For this review, take the finished solid that the model builds, in its own axes (mm). Give positions to 0.01 mm unless a question says otherwise; leave off trailing zeros. Loops run counter-clockwise (first coordinate to the right, second up) from the corner with the lowest first, then second, coordinate; pieces in that order, holes last.
Autodesk Inventor part; units mm, degrees
ref_plane "YZ Plane" through (0, 0, 0) normal (1, 0, 0) x (0, 1, 0)
ref_plane "XZ Plane" through (0, 0, 0) normal (0, 1, 0) x (-1, 0, 0)
ref_plane "XY Plane" through (0, 0, 0) normal (0, 0, 1) x (1, 0, 0)
sketch "スケッチ1" plane through (0, 0, 0) normal (0, 0, 1) x (1, 0, 0)
  line L0 (-70, 75) -> (70, 75)
  line L1 (70, 75) -> (70, -75)
  line L2 (70, -75) -> (-70, -75)
  line L3 (-70, -75) -> (-70, 75)
  line L4 (70, 92.6777) -> (87.6777, 75)
  line L5 (87.6777, 75) -> (70, 57.3223)
  line L6 (70, 57.3223) -> (52.3223, 75)
  line L7 (52.3223, 75) -> (70, 92.6777)
  line L8 (70, -57.3223) -> (87.6777, -75)
  line L9 (87.6777, -75) -> (70, -92.6777)
  line L10 (70, -92.6777) -> (52.3223, -75)
  line L11 (52.3223, -75) -> (70, -57.3223)
  line L12 (-70, -57.3223) -> (-52.3223, -75)
  line L13 (-52.3223, -75) -> (-70, -92.6777)
  line L14 (-70, -92.6777) -> (-87.6777, -75)
  line L15 (-87.6777, -75) -> (-70, -57.3223)
  line L16 (-70, 92.6777) -> (-52.3223, 75)
  line L17 (-52.3223, 75) -> (-70, 57.3223)
  line L18 (-70, 57.3223) -> (-87.6777, 75)
  line L19 (-87.6777, 75) -> (-70, 92.6777)
  point P0 (0, 0)
  point P1 (70, 75)
  dimension "d0" = 150
  dimension "d1" = 75
  dimension "d2" = 140
  dimension "d3" = 70
  dimension "d4" = 12.5
  dimension "d5" = 12.5
  dimension "d6" = 12.5
  dimension "d7" = 12.5
extrude "押し出し1" add sketch "スケッチ1" along normal blind 3
sketch "スケッチ2" plane through (0, 0, 3) normal (0, 0, 1) x (1, 0, 0)
  line L0 (87.6777, 75) -> (70, 57.3223)
  line L1 (70, 92.6777) -> (87.6777, 75)
  line L2 (52.3223, 75) -> (70, 92.6777)
  line L3 (-70, 92.6777) -> (-52.3223, 75)
  line L4 (-87.6777, 75) -> (-70, 92.6777)
  line L5 (-70, 57.3223) -> (-87.6777, 75)
  line L6 (-87.6777, -75) -> (-70, -57.3223)
  line L7 (-70, -92.6777) -> (-87.6777, -75)
  line L8 (-52.3223, -75) -> (-70, -92.6777)
  line L9 (70, -92.6777) -> (52.3223, -75)
  line L10 (87.6777, -75) -> (70, -92.6777)
  line L11 (70, -57.3223) -> (87.6777, -75)
  circle A0 centre (-56.2114, -49.8977) radius 1.5
  circle A1 centre (-44.8977, -61.2114) radius 1.5
  circle A2 centre (44.8977, -61.2114) radius 1.5
  circle A3 centre (56.2114, -49.8977) radius 1.5
  circle A4 centre (56.2114, 49.8977) radius 1.5
  circle A5 centre (44.8977, 61.2114) radius 1.5
  circle A6 centre (-44.8977, 61.2114) radius 1.5
  circle A7 centre (-56.2114, 49.8977) radius 1.5
  point P0 (0, 0)
  dimension "d10" = 3
  dimension "d12" = 40
  dimension "d13" = 40
  dimension "d14" = 4.5
  dimension "d15" = 4.5
  dimension "d16" = 40
  dimension "d17" = 40
  dimension "d18" = 40
  dimension "d19" = 40
  dimension "d20" = 40
  dimension "d21" = 40
  dimension "d22" = 4.5
  dimension "d23" = 4.5
  dimension "d24" = 4.5
  dimension "d25" = 4.5
  dimension "d26" = 4.5
  dimension "d27" = 4.5
hole "穴1" at (44.8977, -61.2114, 3) at (56.2114, -49.8977, 3) at (-44.8977, -61.2114, 3) at (-56.2114, -49.8977, 3) at (44.8977, 61.2114, 3) at (56.2114, 49.8977, 3) at (-56.2114, 49.8977, 3) at (-44.8977, 61.2114, 3) direction (0, 0, -1) diameter 3 end through all
sketch "スケッチ3" plane through (0, 0, 3) normal (0, 0, 1) x (1, 0, 0)
  line L0 (87.6777, 75) -> (70, 57.3223)
  line L1 (70, 92.6777) -> (87.6777, 75)
  line L2 (52.3223, 75) -> (70, 92.6777)
  line L3 (-70, 92.6777) -> (-52.3223, 75)
  line L4 (-87.6777, 75) -> (-70, 92.6777)
  line L5 (-70, 57.3223) -> (-87.6777, 75)
  line L6 (-87.6777, -75) -> (-70, -57.3223)
  line L7 (-70, -92.6777) -> (-87.6777, -75)
  line L8 (-52.3223, -75) -> (-70, -92.6777)
  line L9 (70, -92.6777) -> (52.3223, -75)
  line L10 (87.6777, -75) -> (70, -92.6777)
  line L11 (70, -57.3223) -> (87.6777, -75)
  circle A0 centre (-49.1403, 65.4541) radius 2.25
  circle A1 centre (-60.4541, 54.1403) radius 2.25
  circle A2 centre (-60.4541, -54.1403) radius 2.25
  circle A3 centre (-49.1403, -65.4541) radius 2.25
  circle A4 centre (49.1403, -65.4541) radius 2.25
  circle A5 centre (60.4541, -54.1403) radius 2.25
  circle A6 centre (60.4541, 54.1403) radius 2.25
  circle A7 centre (49.1403, 65.4541) radius 2.25
  point P0 (0, 0)
  dimension "d35" = 4.5
  dimension "d37" = 4.5
  dimension "d38" = 4.5
  dimension "d39" = 34
  dimension "d40" = 34
  dimension "d41" = 4.5
  dimension "d42" = 4.5
  dimension "d43" = 34
  dimension "d44" = 34
  dimension "d45" = 34
  dimension "d46" = 4.5
  dimension "d47" = 4.5
  dimension "d48" = 34
  dimension "d49" = 34
  dimension "d50" = 34
  dimension "d51" = 4.5
  dimension "d52" = 4.5
hole "穴2" at (-60.4541, -54.1403, 3) at (-49.1403, -65.4541, 3) at (49.1403, 65.4541, 3) at (60.4541, 54.1403, 3) at (-60.4541, 54.1403, 3) at (-49.1403, 65.4541, 3) at (49.1403, -65.4541, 3) at (60.4541, -54.1403, 3) direction (0, 0, -1) diameter 4.5 end through all
sketch "スケッチ4" plane through (0, 0, 3) normal (0, 0, 1) x (1, 0, 0)
  line L0 (87.6777, 75) -> (70, 57.3223)
  line L1 (70, 92.6777) -> (87.6777, 75)
  line L2 (52.3223, 75) -> (70, 92.6777)
  line L3 (-70, 92.6777) -> (-52.3223, 75)
  line L4 (-87.6777, 75) -> (-70, 92.6777)
  line L5 (-70, 57.3223) -> (-87.6777, 75)
  line L6 (-87.6777, -75) -> (-70, -57.3223)
  line L7 (-70, -92.6777) -> (-87.6777, -75)
  line L8 (-52.3223, -75) -> (-70, -92.6777)
  line L9 (70, -92.6777) -> (52.3223, -75)
  line L10 (87.6777, -75) -> (70, -92.6777)
  line L11 (70, -57.3223) -> (87.6777, -75)
  line L12 (-70, -57.3223) -> (-52.3223, -75)
  line L13 (52.3223, -75) -> (70, -57.3223)
  line L14 (52.3223, 75) -> (70, 57.3223)
  line L15 (-70, 57.3223) -> (-52.3223, 75)
  point P0 (0, 0)
  dimension "d60" = 25
  dimension "d61" = 25
  dimension "d62" = 25
  dimension "d63" = 25
extrude "押し出し2" cut sketch "スケッチ4" against normal blind 3
sketch "スケッチ6" plane through (-52.3223, 75, 0) normal (0, 1, 0) x (1, 0, 0)
  line L0 (104.6447, 0) -> (0, 0)
  line L1 (0, -3) -> (104.6447, -3)
  line L2 (39.8223, 0) -> (64.8223, 0)
  line L3 (64.8223, 0) -> (64.8223, -3)
  line L4 (64.8223, -3) -> (39.8223, -3)
  line L5 (39.8223, -3) -> (39.8223, 0)
  point P0 (52.3223, 0)
  dimension "d66" = 25
  dimension "d68" = 12.5
extrude "押し出し3" add sketch "スケッチ6" along normal blind 10
sketch "スケッチ7" plane through (0, 0, 3) normal (0, 0, 1) x (1, 0, 0)
  line L0 (-12.5, 85) -> (12.5, 85)
  line L1 (-12.5, 75) -> (-12.5, 85)
  circle A0 centre (-8, 73) radius 1.5
  circle A1 centre (8, 73) radius 1.5
  point P0 (0, 0)
  dimension "d71" = 16
  dimension "d72" = 12
  dimension "d73" = 12
  dimension "d74" = 3
  dimension "d75" = 4.5
hole "穴3" at (-8, 73, 3) at (8, 73, 3) direction (0, 0, -1) diameter 3 end through all
sketch "スケッチ9" plane through (0, 0, 3) normal (0, 0, 1) x (1, 0, 0)
  line L0 (52.3223, -75) -> (-52.3223, -75)
  circle A0 centre (-32.5, -61.5) radius 1.5
  circle A1 centre (-32.5, -28.5) radius 1.5
  circle A2 centre (-32.5, 4.5) radius 1.5
  circle A3 centre (32.5, -61.5) radius 1.5
  circle A4 centre (32.5, -28.5) radius 1.5
  circle A5 centre (32.5, 4.5) radius 1.5
  point P0 (0, 0)
  dimension "d95" = 3
  dimension "d97" = 13.5
  dimension "d98" = 33
  dimension "d99" = 33
  dimension "d100" = 33
  dimension "d101" = 33
  dimension "d102" = 13.5
  dimension "d103" = 65
  dimension "d104" = 65
  dimension "d105" = 65
  dimension "d106" = 32.5
  dimension "d107" = 32.5
  dimension "d108" = 32.5
hole "穴5" at (-32.5, 4.5, 3) at (-32.5, -28.5, 3) at (-32.5, -61.5, 3) at (32.5, -61.5, 3) at (32.5, -28.5, 3) at (32.5, 4.5, 3) direction (0, 0, -1) diameter 3 end through all
equation "\"d33\" = d26"
equation "\"d58\" = d46"
properties material "アルミニウム 6061"
Item 1: The part is to be moulded in two halves that separate along Y. For faces 1 (the flat face through (-1, 6, 3)), 2 (the cylindrical face through (47.24, -66.66, 1.48)), 3 (the flat face through (61.04, -66.28, 1.52)), say which applies: released by +Y, released by -Y, zero draft, split by the parting line, or undercut.
Answer:
face 1: zero draft
face 2: undercut
face 3: released by -Y
Item 2: Take a section at C-C on z = 1.4. State how many separate pieces and enclosed holes the cut face has, and give its area (3 significant figures).
Answer:
separate pieces: 1
enclosed holes: 24
area: 20,400 mm2
Item 3: Take a section at A-A on y = -54.5. Give the boundary of the cut face in (x, z), and give its area (3 significant figures).
Answer:
outline: (-70, 0) - (-62.68, 0) - (-62.68, 3) - (-70, 3) - close; (-58.23, 0) - (58.23, 0) - (58.23, 3) - (-58.23, 3) - close; (62.68, 0) - (70, 0) - (70, 3) - (62.68, 3) - close
area: 393 mm2
Item 4: Clearance check with flat-ended pins moving along their axes: pin 1 Ø1.5 at (x, z) = (36.5, 1) entering from +Y; pin 2 Ø1.5 at (x, z) = (55.5, 2.5) entering from -Y. State where each tip first meets the part, or that it passes through.
Answer:
pin 1: stops at y = 75
pin 2: stops at y = -72.57
Item 5: For L1, parallel to Y at x = 32.5, z = 2.1; L2, parallel to Y at x = -49, z = 2.2; L3, parallel to X at y = 73, z = 1.6, list the stretches that pass through material, from the lowest coordinate up.
Answer:
L1: y = -75 to -63, -60 to -30, -27 to 3, 6 to 75
L2: y = -75 to -67.7, -63.21 to 63.21, 67.7 to 75
L3: x = -54.32 to -9.5, -6.5 to 6.5, 9.5 to 54.32
Item 6: Take a section at B-B on x = -16. Give the boundary of the cut face in (y, z).
Answer:
outline: (-75, 0) - (75, 0) - (75, 3) - (-75, 3) - close
